Design review of the part built by this model. Coordinates are the model's own, in mm. A direction names the side the tool comes from. Give positions to 0.01 mm unless a question says otherwise; leave off trailing zeros. Write each loop counter-clockwise with the first axis right and the second up, starting at its lowest first coordinate (ties: lowest second). Pieces come first, ordered by that corner, then holes. Notation, with made-up numbers: M -29,30 L 18,30 A17 ccw 18,47 Z; hole C 31,36.5 d2. An arc over 180 degrees is marked long. Answer in a Markdown table with one row per item.
```python
from build123d import *

# Parameters (mm, degrees)
SKETCH2_R           = 17.5
BOSS_EXTRUDE1_DEPTH = 181
SKETCH3_R           = 5
CUT_EXTRUDE1_DEPTH  = 181
SKETCH4_R           = 7.5
CUT_EXTRUDE2_DEPTH  = 20
SKETCH5_R           = 12.5
CUT_EXTRUDE3_DEPTH  = 20


with BuildPart() as part:
    # Sketch2 → Boss-Extrude1 (new body)
    with BuildSketch(Plane(origin=(0, 0, 0), x_dir=(0, 0, -1), z_dir=(1, 0, 0))):
        Circle(SKETCH2_R)
    extrude(amount=BOSS_EXTRUDE1_DEPTH)

    # Sketch3 → Cut-Extrude1 (cut)
    with BuildSketch(Plane.XY.offset(17.5)):
        with Locations((20, 0)):
            Circle(SKETCH3_R)
    extrude(amount=-CUT_EXTRUDE1_DEPTH, mode=Mode.SUBTRACT)

    # Sketch4 → Cut-Extrude2 (cut)
    with BuildSketch(Plane(origin=(181, 0, 0), x_dir=(0, 0, -1), z_dir=(1, 0, 0))):
        Circle(SKETCH4_R)
    extrude(amount=-CUT_EXTRUDE2_DEPTH, mode=Mode.SUBTRACT)

    # Sketch5 → Cut-Extrude3 (cut)
    with BuildSketch(Plane(origin=(161, 0, 0), x_dir=(0, 0, -1), z_dir=(1, 0, 0))):
        Circle(SKETCH5_R)
    extrude(amount=-CUT_EXTRUDE3_DEPTH, mode=Mode.SUBTRACT)


solid = part.part
```
1) Add section D-D (x = 20). Write out the cut boundary in (y, z).
Geometry says:
| item | result |
|---|---|
| outline | M -5,-16.77 L -5,16.77 A17.5 ccw Z; M 5,-16.77 A17.5 ccw 5,16.77 Z |
2) Add section A-A (y = 0). Write out the cut boundary in (x, z), and give its area (4 significant figures).
Geometry says:
| item | result |
|---|---|
| outline | M 0,-17.5 L 15,-17.5 L 15,17.5 L 0,17.5 Z; M 25,-17.5 L 181,-17.5 L 181,-7.5 L 161,-7.5 L 161,-12.5 L 141,-12.5 L 141,12.5 L 161,12.5 L 161,7.5 L 181,7.5 L 181,17.5 L 25,17.5 Z |
| area | 5,185 mm^2 |
3) Add section C-C (z = 0). Write out the cut boundary in (x, y), and give its area (3 significant figures).
Geometry says:
| item | result |
|---|---|
| outline | M 0,-17.5 L 181,-17.5 L 181,-7.5 L 161,-7.5 L 161,-12.5 L 141,-12.5 L 141,12.5 L 161,12.5 L 161,7.5 L 181,7.5 L 181,17.5 L 0,17.5 Z; hole C 20,0 d10 |
| area | 5,460 mm^2 |
4) For faces 4 (the face through (151.14, 3.755, -11.923)), 5 (the face through (171.14, 0.33, 7.493)), 6 (the face through (0, 0, 0)), list the 3-axis set-ups (+Z, -Z, +X, -X, +Y, -Y) from which the entire face can be reached by the end or side of a thin tool; tool diameter is ignored.
Geometry says:
| item | result |
|---|---|
| face 4 | none |
| face 5 | +X |
| face 6 | +Z, -Z, -X, +Y, -Y |
5) Add section B-B (z = -10.5). Write out the cut boundary in (x, y), and give its area (3 significant figures).
Geometry says:
| item | result |
|---|---|
| outline | M 0,-14 L 181,-14 L 181,14 L 0,14 Z; hole C 20,0 d10; hole M 141,-6.78 L 161,-6.78 L 161,6.78 L 141,6.78 Z |
| area | 4,720 mm^2 |
6) To check wall thickness, follow probe 1 along Y at (x, z) = (147.5, -0.5); probe 2 along X at (y, z) = (10, 1); probe 3 along Y at (x, z) = (176.5, 0). State the ranges of each line that lie inside material, in increasing order. Write a range as [from, to].
Geometry says:
| item | result |
|---|---|
| probe 1 | [-17.49, -12.49], [12.49, 17.49] |
| probe 2 | [0, 141], [161, 181] |
| probe 3 | [-17.5, -7.5], [7.5, 17.5] |
7) The part is to be moulded in two halves that separate along Z. For faces 1 (the face through (141, 0, 0)), 2 (the face through (89.233, -10.648, 13.887)), 3 (the face through (15, 0, 0)), say which applies: released by +Z, released by -Z, zero draft, split by the parting line, or undercut.
Geometry says:
| item | result |
|---|---|
| face 1 | undercut |
| face 2 | split by the parting line |
| face 3 | zero draft |
8) Insertion check: P1, Ø2, axis at x = 110, z = -8.5, coming from the -Y side; P2, Ø2, axis at x = 81, y = -2.5, coming from the +Z side; P3, Ø8, axis at x = 29.5, y = 9.5, coming from the +Z side; P4, Ø9, axis at x = 20, y = 0, coming from the +Z side. Each pin has a flat end and moves straight along its axis. Give the tip position at first contact, or say it passes through.
Geometry says:
| item | result |
|---|---|
| P1 | y = -15.81 |
| P2 | z = 17.44 |
| P3 | z = 16.61 |
| P4 | through |
